Check sheet for the modelled part. Datum: model origin and axes. Units: mm. Face numbers are marked on the shaded views. Coordinates: 2 decimals unless noted, no trailing zeros. Loops run counter-clockwise (first coordinate to the right, second up) from the corner with the lowest first, then second, coordinate; pieces in that order, holes last. Notation, with made-up numbers: (25.5, 19.25) - (31.5, 19.25) arc R17 cw to (31.5, 27.25) - close; hole circle Ø11 at (60, -8). An arc over 180 degrees is marked (long way). Write each question's results on one line, items separated by ' | '. Start each with the question number.
1. Draft check along X on the marked faces 1, 2, 3 and 4. Enter one of: released by +X, released by -X, zero draft, split by the parting line, or undercut.
2. Cross-section at D-D (x = -8). Record the cut outline in (y, z), and give its area (3 significant figures).
3. Thickness scan on line 1 (Y direction, x = 0, z = 0.3) (3 decimals); line 2 (X direction, y = 50, z = -8); line 3 (Y direction, x = 20, z = -42). Record the ranges inside material, lowest first. Write a range as [from, to].
4. Gauge pin test, flat ends, axial feed: P1, Ø9.5, axis at x = 0, z = -4.75, coming from the +Y side; P2, Ø11.5, axis at x = -15, z = -55.5, coming from the +Y side; P3, Ø20, axis at x = 0, y = 90, coming from the -Z side; P4, Ø5, axis at x = 15, z = -55.5, coming from the +Y side. Record the tip position at first contact, or that the pin passes through.
5. Cross-section at B-B (y = 110). Record the cut outline in (x, z) (3 decimals).
6. Cross-section at A-A (z = -24.75). Record the cut outline in (x, y), and give its area (3 significant figures).
7. Cross-section at C-C (y = 80). Record the cut outline in (x, z), and give its area (3 significant figures).
```python
from build123d import *

# Parameters (mm, degrees)
SKETCH_1_R             = 25
SKETCH_1_R_2           = 11
SKETCH_1_R_3           = 2.05
EXTRUDE_1_DEPTH        = 1.5
EXTRUDE_START          = -3
EXTRUDE_2_DEPTH        = 3
SKETCH_4_W             = 50
SKETCH_4_H             = 3
EXTRUDE_3_DEPTH        = 65
CUT_EXTRUDE_1_DEPTH    = 55
SKETCH_7_R             = 2.1
CUT_EXTRUDE_2_DEPTH    = 55
SKETCH_9_R             = 3.625
CUT_EXTRUDE_3_DEPTH    = 1.5
CUT_EXTRUDE_START      = -1.5
SKETCH_11_R            = 3.625
SKETCH_11_R_2          = 2.05
CUT_EXTRUDE_4_DEPTH    = 1.5
SKETCH_12_R            = 1.55
SKETCH_12_R_2          = 5
CUT_EXTRUDE_5_DEPTH    = 6.5
CUT_EXTRUDE_START_2    = -1
SKETCH_13_R            = 3
SKETCH_13_R_2          = 1.55
CUT_EXTRUDE_13_DEPTH   = 1
EXTRUDE_4_DEPTH        = 2
FILLET_1_R             = 4
FILLET_1_OF_MIRROR_1_R = 4


with BuildPart() as part:
    # 草图1 → 凸台-拉伸1 (new, symmetric)
    with BuildSketch(Plane.XY):
        with Locations((0, 90)):
            Circle(SKETCH_1_R)
        with Locations((0, 90)):
            Circle(SKETCH_1_R_2, mode=Mode.SUBTRACT)
        with Locations((0, 110)):
            Circle(SKETCH_1_R_3, mode=Mode.SUBTRACT)
        with Locations((17.320508076, 80)):
            Circle(SKETCH_1_R_3, mode=Mode.SUBTRACT)
        with Locations((-17.320508076, 80)):
            Circle(SKETCH_1_R_3, mode=Mode.SUBTRACT)
    extrude(amount=EXTRUDE_1_DEPTH, both=True)

    # 草图3 → 凸台-拉伸2 (add)
    with BuildSketch(Plane(origin=(0, 0, -1.5), x_dir=(-1, 0, 0), z_dir=(0, 0, -1)).offset(EXTRUDE_START)):
        with BuildLine():
            ThreePointArc((25, 90), (0, 65), (-25, 90))
            Line((-25, 90), (-25, 52.5))
            Line((-25, 52.5), (25, 52.5))
            Line((25, 52.5), (25, 90))
        make_face()
    extrude(amount=EXTRUDE_2_DEPTH)

    # 草图4 → 凸台-拉伸3 (add)
    with BuildSketch(Plane.XY.offset(1.5)):
        with Locations((0, 51)):
            Rectangle(SKETCH_4_W, SKETCH_4_H)
    extrude(amount=-EXTRUDE_3_DEPTH)

    # 草图6 → 切除-拉伸1 (cut)
    with BuildSketch(Plane(origin=(0, 52.5, 0), x_dir=(1, 0, 0), z_dir=(0, 1, 0))):
        Polygon((-25, 53.5), (-15, 63.5), (-25, 63.5), align=None)
        Polygon((25, 63.5), (15, 63.5), (25, 53.5), align=None)
    extrude(amount=-CUT_EXTRUDE_1_DEPTH, mode=Mode.SUBTRACT)

    # 草图7 → 切除-拉伸2 (cut)
    with BuildSketch(Plane(origin=(0, 52.5, 0), x_dir=(1, 0, 0), z_dir=(0, 1, 0))):
        with Locations(Location((-15, 55.5, 0), (0, 0, 270))):
            Circle(SKETCH_7_R)
        with Locations(Location((15, 55.5, 0), (0, 0, 270))):
            Circle(SKETCH_7_R)
        with Locations(Location((15, 8, 0), (0, 0, 270))):
            Circle(SKETCH_7_R)
        with Locations(Location((-15, 8, 0), (0, 0, 270))):
            Circle(SKETCH_7_R)
    extrude(amount=-CUT_EXTRUDE_2_DEPTH, mode=Mode.SUBTRACT)

    # 草图9 → 切除-拉伸3 (cut)
    with BuildSketch(Plane(origin=(0, 52.5, 0), x_dir=(1, 0, 0), z_dir=(0, 1, 0))):
        with Locations(Location((-15, 55.5, 0), (0, 0, 270))):
            Circle(SKETCH_9_R)
        with Locations(Location((15, 55.5, 0), (0, 0, 270))):
            Circle(SKETCH_9_R)
        with Locations(Location((15, 8, 0), (0, 0, 270))):
            Circle(SKETCH_9_R)
        with Locations(Location((-15, 8, 0), (0, 0, 270))):
            Circle(SKETCH_9_R)
    extrude(amount=-CUT_EXTRUDE_3_DEPTH, mode=Mode.SUBTRACT)

    # 草图11 → 切除-拉伸4 (cut)
    # profile 1 of 3: a face of its own
    with BuildSketch(Plane.XY.offset(1.5).offset(CUT_EXTRUDE_START)):
        with Locations((0, 110)):
            Circle(SKETCH_11_R)
        with Locations((0, 110)):
            Circle(SKETCH_11_R_2, mode=Mode.SUBTRACT)
    # profile 2 of 3: a face of its own
    with BuildSketch(Plane.XY.offset(1.5).offset(CUT_EXTRUDE_START)):
        with Locations((17.320508076, 80)):
            Circle(SKETCH_11_R)
        with Locations((17.320508076, 80)):
            Circle(SKETCH_11_R_2, mode=Mode.SUBTRACT)
    # profile 3 of 3: a face of its own
    with BuildSketch(Plane.XY.offset(1.5).offset(CUT_EXTRUDE_START)):
        with Locations((-17.320508076, 80)):
            Circle(SKETCH_11_R)
        with Locations((-17.320508076, 80)):
            Circle(SKETCH_11_R_2, mode=Mode.SUBTRACT)
    extrude(amount=CUT_EXTRUDE_4_DEPTH, mode=Mode.SUBTRACT)

    # 草图12 → 切除-拉伸5 (cut)
    with BuildSketch(Plane.XZ.offset(-49.5)):
        with Locations((0, -4.75)):
            Circle(SKETCH_12_R)
        with Locations((0, -44.75)):
            Circle(SKETCH_12_R)
        with Locations((0, -24.75)):
            Circle(SKETCH_12_R_2)
    extrude(amount=-CUT_EXTRUDE_5_DEPTH, mode=Mode.SUBTRACT)

    # 草图13 → 切除-拉伸13 (cut)
    # profile 1 of 2: a face of its own
    with BuildSketch(Plane(origin=(0, 52.5, 0), x_dir=(1, 0, 0), z_dir=(0, 1, 0)).offset(CUT_EXTRUDE_START_2)):
        with Locations(Location((0, 4.75, 0), (0, 0, 270))):
            Circle(SKETCH_13_R)
        with Locations((0, 4.75)):
            Circle(SKETCH_13_R_2, mode=Mode.SUBTRACT)
    # profile 2 of 2: a face of its own
    with BuildSketch(Plane(origin=(0, 52.5, 0), x_dir=(1, 0, 0), z_dir=(0, 1, 0)).offset(CUT_EXTRUDE_START_2)):
        with Locations(Location((0, 44.75, 0), (0, 0, 270))):
            Circle(SKETCH_13_R)
        with Locations((0, 44.75)):
            Circle(SKETCH_13_R_2, mode=Mode.SUBTRACT)
    extrude(amount=CUT_EXTRUDE_13_DEPTH, mode=Mode.SUBTRACT)

    # 草图14 → 凸台-拉伸4 (add)
    with BuildSketch(Plane(origin=(25, 0, 0), x_dir=(0, 0, -1), z_dir=(1, 0, 0))):
        Polygon((1.5, 61), (10, 52.5), (1.5, 52.5), align=None)
    extrude_4 = extrude(amount=-EXTRUDE_4_DEPTH)

    # 圆角1
    fillet_1_edges = [part.edges().sort_by_distance(p)[0] for p in [
        (24, 61, -1.5),
        (24, 52.5, -10),
    ]]
    fillet(fillet_1_edges, radius=FILLET_1_R)

    # 镜向1: 凸台-拉伸4 across plane
    add(extrude_4.mirror(Plane(origin=(0, 0, 0), x_dir=(0, 0, 1), z_dir=(1, 0, 0))))

    # 圆角1 of 镜向1
    fillet_1_of_mirror_1_edges = [part.edges().sort_by_distance(p)[0] for p in [
        (-24, 61, -1.5),
        (-24, 52.5, -10),
    ]]
    fillet(fillet_1_of_mirror_1_edges, radius=FILLET_1_OF_MIRROR_1_R)


solid = part.part
```
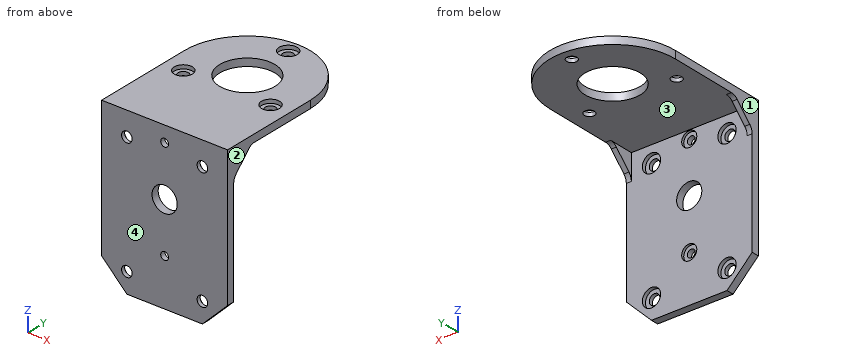
Established:
1) face 1: released by -X | face 2: released by +X | face 3: undercut | face 4: zero draft
2) outline: (49.5, -63.5) - (52.5, -63.5) - (52.5, -1.5) - (82.45, -1.5) - (82.45, 1.5) - (49.5, 1.5) - close; (97.55, -1.5) - (113.69, -1.5) - (113.69, 1.5) - (97.55, 1.5) - close | area: 333 mm^2
3) line 1: [49.5, 79], [101, 106.375], [113.625, 115] | line 2: [-25, -17.1], [-12.9, 12.9], [17.1, 25] | line 3: [49.5, 52.5]
4) P1: y = 115 | P2: y = 52.5 | P3: through | P4: y = 51
5) outline: (-15, -1.5) - (-2.05, -1.5) - (-2.05, 0) - (-3.625, 0) - (-3.625, 1.5) - (-15, 1.5) - close; (2.05, -1.5) - (15, -1.5) - (15, 1.5) - (3.625, 1.5) - (3.625, 0) - (2.05, 0) - close
6) outline: (-25, 49.5) - (-5, 49.5) - (-5, 52.5) - (-25, 52.5) - close; (5, 49.5) - (25, 49.5) - (25, 52.5) - (5, 52.5) - close | area: 120 mm^2
7) outline: (-25, -1.5) - (-19.37, -1.5) - (-19.37, 0) - (-20.95, 0) - (-20.95, 1.5) - (-25, 1.5) - close; (-15.27, -1.5) - (-4.58, -1.5) - (-4.58, 1.5) - (-13.7, 1.5) - (-13.7, 0) - (-15.27, 0) - close; (4.58, -1.5) - (15.27, -1.5) - (15.27, 0) - (13.7, 0) - (13.7, 1.5) - (4.58, 1.5) - close; (19.37, -1.5) - (25, -1.5) - (25, 1.5) - (20.95, 1.5) - (20.95, 0) - (19.37, 0) - close | area: 88.5 mm^2
